For this review, take the finished solid that the model builds, in its own axes (mm). A direction names the side the tool comes from. Give positions to 0.01 mm unless a question says otherwise; leave off trailing zeros. Write each loop counter-clockwise with the first axis right and the second up, starting at its lowest first coordinate (ties: lowest second). Pieces come first, ordered by that corner, then holes. Notation, with made-up numbers: (34.5, 40.5) -> (56.5, 40.5) arc R27 cw to (56.5, 77.5) -> close; hole circle Ø9 at (-15.5, 22.25). An arc over 180 degrees is marked (long way). Write item = value, one per line.
```python
from build123d import *

# Parameters (mm, degrees)
BOSS_EXTRUDE1_DEPTH      = 91.992761
BOSS_EXTRUDE1_DEPTH_BACK = 12.782239
BOSS_EXTRUDE2_DEPTH      = 93.6375
CUT_EXTRUDE1_DEPTH       = 144.067335103
FILLET1_R                = 5


with BuildPart() as part:
    # Sketch1 → Boss-Extrude1 (new, two sides: drawn at the far end of the back side and taken through both)
    with BuildSketch(Plane.XY.offset(-BOSS_EXTRUDE1_DEPTH_BACK)):
        Polygon((-68.287510941, 96.719618957), (-66.487510941, 98.519618957), (-64.787510941, 98.519618957), (-64.787510941, 14.882118957), (-66.487510941, 14.882118957), (-68.287510941, 16.682118957), (-71.823044847, 13.146585051), (-68.558578753, 9.882118957), (-54.787510941, 9.882118957), (-54.787510941, 103.519618957), (-68.558578753, 103.519618957), (-71.823044847, 100.255152863), align=None)
    extrude(amount=BOSS_EXTRUDE1_DEPTH + BOSS_EXTRUDE1_DEPTH_BACK)

    # Sketch2 → Boss-Extrude2 (add)
    with BuildSketch(Plane(origin=(0, 9.882118957, 0), x_dir=(1, 0, 0), z_dir=(0, 1, 0))):
        Polygon((-54.787510941, 12.782239353), (-54.787510941, -91.992760647), (-28.880926753, 5.928233091), align=None)
    extrude(amount=BOSS_EXTRUDE2_DEPTH)

    # Sketch3 → Cut-Extrude1 (cut, through all)
    with BuildSketch(Plane.ZY.offset(64.787510941)):
        with BuildLine():
            Line((49.974010647, 92.719618957), (-12.782239353, 92.719618957))
            Line((-12.782239353, 92.719618957), (-12.782239353, 20.682118957))
            Line((-12.782239353, 20.682118957), (49.974010647, 20.682118957))
            ThreePointArc((49.974010647, 20.682118957), (85.992760647, 56.700868957), (49.974010647, 92.719618957))
        make_face()
        with BuildLine():
            Line((91.543139818, 20.882118957), (97.180187327, 20.882118957))
            Line((97.180187327, 20.882118957), (97.180187327, 92.519618957))
            Line((97.180187327, 92.519618957), (91.543139818, 92.519618957))
            ThreePointArc((91.543139818, 92.519618957), (84.486417774, 88.288262479), (84.894572363, 80.070287456))
            ThreePointArc((84.894572363, 80.070287456), (91.992760647, 56.700868957), (84.894572363, 33.331450457))
            ThreePointArc((84.894572363, 33.331450457), (84.486417774, 25.113475435), (91.543139818, 20.882118957))
        make_face()
    extrude(amount=-CUT_EXTRUDE1_DEPTH, mode=Mode.SUBTRACT)

    # Fillet1
    fillet1_edges = [part.edges().sort_by_distance(p)[0] for p in [
        (-54.787510941, 15.282118957, -12.782239),
        (-54.787510941, 98.119618957, -12.782239),
        (-28.880926753, 15.282118957, -5.928233091),
        (-28.880926753, 98.119618957, -5.928233091),
        (-54.787510941, 15.382118957, 91.992761),
        (-54.787510941, 98.019618957, 91.992761),
    ]]
    fillet(fillet1_edges, radius=FILLET1_R)


solid = part.part
```
(1) Tool access review of faces 1 (the face through (-58.7, 25.22, 84.43)), 2 (the face through (-52, 20.682, 18)), 3 (the face through (-55.55, 15.814, 90.927)), 4 (the face through (-54, 103.52, 27)), 5 (the face through (-70.03, 14.94, 38.87)): name each direction out of +Z, -Z, +X, -X, +Y, -Y from which nothing blocks a thin tool from reaching the whole face with its end or side.
Answers below:
face_1 = +Z, +X, -X
face_2 = -Z, +X, -X
face_3 = +Z, +X, -Y
face_4 = +Z, -Z, +X, -X, +Y
face_5 = +Z, -Z, -X
(2) Take a section at A-A (z = 20.5). Write out the cut boundary in (x, y).
Answers below:
outline = (-71.82, 13.15) -> (-68.56, 9.88) -> (-35.87, 9.88) -> (-35.87, 20.68) -> (-64.79, 20.68) -> (-64.79, 14.88) -> (-66.49, 14.88) -> (-68.29, 16.68) -> close; (-71.82, 100.26) -> (-68.29, 96.72) -> (-66.49, 98.52) -> (-64.79, 98.52) -> (-64.79, 92.72) -> (-35.87, 92.72) -> (-35.87, 103.52) -> (-68.56, 103.52) -> close
(3) Take a section at C-C (z = 73). Write out the cut boundary in (x, y), plus the area to 3 significant figures.
Answers below:
outline = (-71.82, 13.15) -> (-68.56, 9.88) -> (-49.76, 9.88) -> (-49.76, 29) -> (-64.79, 29) -> (-64.79, 14.88) -> (-66.49, 14.88) -> (-68.29, 16.68) -> close; (-71.82, 100.26) -> (-68.29, 96.72) -> (-66.49, 98.52) -> (-64.79, 98.52) -> (-64.79, 84.4) -> (-49.76, 84.4) -> (-49.76, 103.52) -> (-68.56, 103.52) -> close
area = 638 mm^2
(4) The part is to be moulded in two halves that separate along X. For faces 6 (the face through (-54, 9.882, 27)), 7 (the face through (-70.08, 98.51, 38.87)), 8 (the face through (-64.788, 60, 86)), say which applies: released by +X, released by -X, zero draft, split by the parting line, or undercut.
Answers below:
face_6 = zero draft
face_7 = released by -X
face_8 = undercut
(5) To check wall thickness, follow probe 1 along Y at (x, z) = (-47.5, 2.5); probe 2 along Y at (x, z) = (-70, -3); probe 3 along X at (y, z) = (15.5, 18). State the ranges of each line that lie inside material, in increasing order.
Answers below:
probe_1 = 9.88 to 20.68, 92.72 to 103.52
probe_2 = 11.32 to 14.97, 98.43 to 102.08
probe_3 = -69.47 to -67.11, -64.79 to -35.21
(6) Take a section at B-B (x = -41). Write out the cut boundary in (y, z).
Answers below:
outline = (9.88, -9.13) -> (20.68, -9.13) -> (20.68, 39.88) -> (9.88, 39.88) -> close; (92.72, -9.13) -> (103.52, -9.13) -> (103.52, 39.88) -> (92.72, 39.88) -> close
(7) For pin 1 (4 mm diameter, centred on x = -65.5, y = 31, fed in from -Z); pin 2 (6 mm diameter, centred on x = -45, z = 76.5, fed in from -Y), all flat-tipped, find the tip position at first contact; note any pin that passes through.
Answers below:
pin_1 = 73.15
pin_2 = through
(8) Take a section at D-D (y = 40.5). Write out the cut boundary in (x, z).
Answers below:
outline = (-64.79, 82.14) -> (-52.18, 82.14) -> (-53.93, 88.74) -> (-64.79, 88.74) -> close
